Verification items for the finished model (mm, model axes). A direction names the side the tool comes from. Coordinates: 2 decimals unless noted, no trailing zeros. Loops run counter-clockwise (first coordinate to the right, second up) from the corner with the lowest first, then second, coordinate; pieces in that order, holes last. Notation, with made-up numbers: (37, 18.5) -> (79, 18.5) arc R17 ccw to (79, 25.5) -> close; hole circle Ø8 at (-21.75, 35.25). An arc over 180 degrees is marked (long way). Answer as a JSON object with one key per item and string values. Group by question number.
Q1. Set-up check for faces 4 (the flat face through (37, 6, -54)), 5 (the flat face through (-18.4, 5.1, -32.1)): record each of +Z, -Z, +X, -X, +Y, -Y from which the full face is reachable in a straight line by a thin tool's end or side.
Q2. Scan lines: L1, parallel to X at y = 0.5, z = -108.5; L2, parallel to X at y = 4.5, z = -45; L3, parallel to Z at x = -53.5, y = 3.75. Record each from-to range of solid material in increasing order.
Q3. Cross-section at D-D on z = -80. Record the boundary of the cut face in (x, y), and give its area (3 significant figures).
Q4. Cross-section at C-C on y = 4. Give the number of separate pieces and of enclosed holes in the cut face, and give its area (3 significant figures).
Q5. Release check for a two-part mould opening along Z. For faces 1 (the flat face through (9.269, 3.042, -6.195)), 2 (the cylindrical face through (48.604, 2.958, -70.189)), 3 (the flat face through (-34, 0, -53)) record: released by +Z, released by -Z, zero draft, split by the parting line, or undercut.
Q6. Gauge pin test, flat ends, axial feed: pin 1 Ø3 at (y, z) = (4.5, -57) entering from -X; pin 2 Ø4 at (x, y) = (24, 4) entering from -Z; pin 3 Ø1 at (x, y) = (-32.5, 4) entering from +Z. Record the tip position at first contact, or that the pin passes through.
Q7. Cross-section at A-A on z = 5. Record the boundary of the cut face in (x, y), and give its area (3 significant figures).
Q8. Cross-section at B-B on x = -35.5. Record the boundary of the cut face in (y, z), and give its area (3 significant figures).
Autodesk Fusion 360 part; units mm, degrees
sketch "Sketch1" plane through (0, 0, 0) normal (0, 1, 0) x (1, 0, 0)
  line L0 (-120, 0) -> (-10, 0)
  line L1 (5, 8.6603) -> (60, 103.923)
  arc A0 (60, 103.923) -> (-120, 0) centre (0, 0) ccw
  arc A1 (5, 8.6603) -> (-10, 0) centre (0, 0) ccw
  dimension "d57" = 240
  dimension "d58" = 120
  dimension "d59" = 20
extrude "Extrude3" add sketch "Sketch1" along normal blind 10
sketch "Sketch9" plane through (0, 0, 0) normal (0, 0, 1) x (1, 0, 0)
  line L0 (-120, 0) -> (-10, 0)
  line L1 (-10, 0) -> (-10, 10)
  line L2 (-10, 10) -> (-120, 10)
  line L3 (-120, 10) -> (-120, 0)
  line L4 (-120, 10) -> (-10, 10)
  line L5 (-10, 10) -> (-10, 6)
  line L6 (-10, 6) -> (-120, 6)
  line L7 (-120, 6) -> (-120, 10)
  dimension "d60" = 4
extrude "Extrude8" add sketch "Sketch9" along normal blind 10 contours L1 L2 L3 L4 L5 L6 L7
sketch "Sketch12" plane through (0, 0, 0) normal (0.866, 0, 0.5) x (0.5, 0, -0.866)
  line L0 (10, 0) -> (120, 0)
  line L1 (120, 0) -> (120, 10)
  line L2 (120, 10) -> (10, 10)
  line L3 (10, 10) -> (10, 0)
  line L4 (10, 0) -> (120, 0)
  line L5 (120, 0) -> (120, 6)
  line L6 (120, 6) -> (10, 6)
  line L7 (10, 6) -> (10, 0)
  dimension "d63" = 6
extrude "Extrude9" add sketch "Sketch12" along normal blind 10 contours L0 L1 L3 L4 L5 L6 L7
sketch "Sketch13" plane through (0, 10, 0) normal (0, 1, 0) x (-1, 0, 0)
  arc A0 (-60, -103.923) -> (120, 0) centre (0, 0) ccw
  line L0 (120, 0) -> (120, 10)
  line L1 (120, 10) -> (10, 10)
  line L2 (10, 10) -> (10, 0)
  arc A1 (-5, -8.6603) -> (10, 0) centre (0, 0) ccw
  line L3 (-5, -8.6603) -> (-60, -103.923)
  point P0 (85, 5)
  point P1 (45, 5)
  dimension "d68" = 35
  dimension "d69" = 35
hole "Hole1" at (-85, 10, 5) at (-45, 10, 5) direction (0, -1, 0) diameter 4 depth 4 tip angle 118 countersink diameter 6 countersink angle 90
sketch "Sketch14" plane through (0, 6, 0) normal (0, 1, 0) x (-1, 0, 0)
  line L0 (-60, -103.923) -> (-5, -8.6603)
  line L1 (-5, -8.6603) -> (-13.6603, -3.6603)
  line L2 (-13.6603, -3.6603) -> (-68.6603, -98.923)
  line L3 (-68.6603, -98.923) -> (-60, -103.923)
  line L4 (-9.3301, -6.1603) -> (-64.3301, -101.423) construction
  point P0 (-26.8301, -36.4711)
  point P1 (-46.8301, -71.1122)
  dimension "d75" = 35
  dimension "d76" = 35
hole "Hole2" at (26.8301, 6, -36.4711) at (46.8301, 6, -71.1122) direction (0, -1, 0) diameter 4 depth 15 tip angle 118
sketch "Sketch15" plane through (0, 10, 0) normal (0, 1, 0) x (-1, 0, 0)
  circle A0 centre (85, 5) radius 3
  circle A1 centre (45, 5) radius 3
  arc A2 (-60, -103.923) -> (120, 0) centre (0, 0) ccw
  line L0 (120, 0) -> (120, 10)
  line L1 (120, 10) -> (10, 10)
  line L2 (10, 10) -> (10, 0)
  arc A3 (-5, -8.6603) -> (10, 0) centre (0, 0) ccw
  line L3 (-5, -8.6603) -> (-60, -103.923)
  line L4 (0, 0) -> (60, -103.923) construction
  line L5 (10, 0) -> (120, 0)
  line L6 (56.6506, -48.1218) -> (13.3494, -73.1218) construction
  line L7 (5.7058, -27.8827) -> (21.2942, -18.8827)
  line L8 (5.7058, -27.8827) -> (10.7058, -36.5429)
  line L9 (10.7058, -36.5429) -> (26.2942, -27.5429)
  line L10 (26.2942, -27.5429) -> (21.2942, -18.8827)
  line L11 (57.1962, -87.0666) -> (46.8038, -93.0666) construction
  dimension "d80" = 60
  dimension "d81" = 50
  dimension "d82" = 25
  dimension "d83" = 50
  dimension "d89" = 43
  dimension "d90" = 9
  dimension "d91" = 18
  dimension "d92" = 10
  dimension "d95" = 6
  dimension "d96" = 12
  dimension "d97" = 34
hole "Hole3" at (-56.6506, 10, -48.1218) at (-13.3494, 10, -73.1218) at (-57.1962, 10, -87.0666) at (-46.8038, 10, -93.0666) direction (0, -1, 0) diameter 3.2 depth 35 tip angle 118 countersink diameter 6 countersink angle 90
extrude "Extrude10" cut sketch "Sketch15" against normal blind 20 contours L7 L8 L9 L10
sketch "Sketch16" plane through (0, 10, 0) normal (0, 1, 0) x (-1, 0, 0)
  line L0 (120, 0) -> (120, 10)
  line L1 (10, 0) -> (10, 10)
  line L2 (-5, -8.6603) -> (-13.6603, -3.6603)
  line L3 (-60, -103.923) -> (-68.6603, -98.923)
  line L4 (120, 5) -> (10, 5) construction
  line L5 (-9.3301, -6.1603) -> (-64.3301, -101.423) construction
  line L6 (-11.0289, -109.1025) -> (-97.6314, -59.1025) construction
  line L7 (100, -45) -> (100, 55) construction
  dimension "d98" = 100
  dimension "d99" = 50
  dimension "d100" = 20
  dimension "d101" = 20
  dimension "d102" = 100
  dimension "d103" = 50
sketch "Sketch17" plane through (0, 0, 0) normal (0, -1, 0) x (1, 0, 0)
  line L0 (-10.7058, -36.5429) -> (-26.2942, -27.5429)
  line L1 (-26.2942, -27.5429) -> (-21.2942, -18.8827)
  line L2 (-21.2942, -18.8827) -> (-5.7058, -27.8827)
  line L3 (-5.7058, -27.8827) -> (-10.7058, -36.5429)
  circle A0 centre (-57.1962, -87.0666) radius 1.6
  circle A1 centre (-56.6506, -48.1218) radius 1.6
  circle A2 centre (-13.3494, -73.1218) radius 1.6
  circle A3 centre (-46.8038, -93.0666) radius 1.6
  circle A4 centre (26.8301, -36.4711) radius 2
  circle A5 centre (46.8301, -71.1122) radius 2
  arc A6 (-120, 0) -> (60, -103.923) centre (0, 0) ccw
  line L4 (60, -103.923) -> (68.6603, -98.923)
  line L5 (68.6603, -98.923) -> (13.6603, -3.6603)
  line L6 (13.6603, -3.6603) -> (5, -8.6603)
  arc A7 (-10, 0) -> (5, -8.6603) centre (0, 0) ccw
  line L7 (-10, 0) -> (-120, 0)
sketch "Sketch18" plane through (0, 0, 0) normal (0, -1, 0) x (1, 0, 0)
  point P0 (-100, -45)
  point P1 (11.0289, -109.1025)
  point P2 (-100, -45)
  point P3 (11.0289, -109.1025)
hole "Hole4" at (-100, 0, -45) at (11.0289, 0, -109.1025) direction (0, 1, 0) diameter 3.2 depth 25 tip angle 180 countersink diameter 6 countersink angle 90
sketch "Sketch19" plane through (0, 10, 0) normal (0, 1, 0) x (-1, 0, 0)
  circle A0 centre (100, -45) radius 1.6
  circle A1 centre (-11.0289, -109.1025) radius 1.6
  line L0 (26.2942, -27.5429) -> (10.7058, -36.5429)
  line L1 (10.7058, -36.5429) -> (5.7058, -27.8827)
  line L2 (5.7058, -27.8827) -> (21.2942, -18.8827)
  line L3 (21.2942, -18.8827) -> (26.2942, -27.5429)
  circle A2 centre (57.1962, -87.0666) radius 3
  circle A3 centre (56.6506, -48.1218) radius 3
  circle A4 centre (13.3494, -73.1218) radius 3
  circle A5 centre (46.8038, -93.0666) radius 3
  circle A6 centre (85, 5) radius 3
  circle A7 centre (45, 5) radius 3
  arc A8 (-60, -103.923) -> (120, 0) centre (0, 0) ccw
  line L4 (120, 0) -> (120, 10)
  line L5 (120, 10) -> (10, 10)
  line L6 (10, 10) -> (10, 0)
  arc A9 (-5, -8.6603) -> (10, 0) centre (0, 0) ccw
  line L7 (-5, -8.6603) -> (-60, -103.923)
  line L8 (5, -8.6603) -> (60, -103.923) construction
  line L9 (91.2096, -77.9796) -> (46.188, 0) construction
  line L10 (21.9275, -117.9796) -> (-23.094, -40) construction
  line L11 (10, 0) -> (120, 0)
  circle A10 centre (86.2096, -69.3193) radius 2
  circle A11 centre (16.9275, -109.3193) radius 2
  circle A12 centre (55, -95.2628) radius 2
  point P0 (120, 5)
  dimension "d111" = 40
  dimension "d112" = 40
  dimension "d113" = 4
  dimension "d114" = 10
  dimension "d115" = 4
  dimension "d116" = 10
  dimension "d117" = 4
  dimension "d118" = 10
extrude "Extrude11" cut sketch "Sketch19" against normal blind 80 contours A10 | A11 | A12
pattern_linear "R-Pattern1" count 6 spacing 13 along (0.5, 0, 0.866) of "Extrude11"
equation "d82 = d81 / 2"
equation "d90 = d91 / 2"
equation "d96 = d95 * 2"
equation "d99 = d98 / 2"
equation "d101 = d100"
equation "d102 = d98"
equation "d103 = d99"
equation "d112 = d111"
equation "d116 = d114"
equation "d118 = d114"
Computed values:
{
 "1": {"face 4": "+Z, +X, +Y", "face 5": "+Y, -Y"},
 "2": {"L1": "x = -51.26 to -18.75, -15.1 to 8.6, 13.46 to 51.26", "L2": "x = -111.24 to -101.6, -98.4 to -74.08, -72.34 to 37.53", "L3": "z = -107.41 to -96.59, -93.94 to -15.02, -11.04 to 0"},
 "3": {"outline": "(-89.44, 0) -> (57.74, 0) -> (57.74, 6) -> (46.19, 6) -> (46.19, 10) -> (-89.44, 10) -> close", "area": "1,430 mm²"},
 "4": {"separate pieces": "1", "enclosed holes": "27", "area": "15,600 mm²"},
 "5": {"face 1": "released by +Z", "face 2": "undercut", "face 3": "zero draft"},
 "6": {"pin 1": "stops at x = -106.39", "pin 2": "stops at z = -117.97", "pin 3": "stops at z = 0"},
 "7": {"outline": "(-120, 6) -> (-87, 6) -> (-87, 9) -> (-88, 10) -> (-120, 10) -> close; (-83, 6) -> (-47, 6) -> (-47, 9) -> (-48, 10) -> (-82, 10) -> (-83, 9) -> close; (-43, 6) -> (-10, 6) -> (-10, 10) -> (-42, 10) -> (-43, 9) -> close", "area": "406 mm²"},
 "8": {"outline": "(0, -114.63) -> (10, -114.63) -> (10, -63.49) -> (0, -63.49) -> close; (0, -59.49) -> (10, -59.49) -> (10, 10) -> (6, 10) -> (6, 0) -> (0, 0) -> close", "area": "1,150 mm²"}
}
